For this review, take the finished solid that the model builds, in its own axes (mm). Face numbers are marked on the shaded views. A direction names the side the tool comes from. Coordinates: 2 decimals unless noted, no trailing zeros. Write each loop counter-clockwise with the first axis right and the second up, starting at its lowest first coordinate (ties: lowest second). Pieces come first, ordered by that corner, then holes. Notation, with made-up numbers: M 0.25,-15.75 L 19.25,-15.75 A31 cw 19.25,9.25 Z; hole C 51.5,-33 d4. An arc over 180 degrees is marked long. Return JSON: item names as keys, results as strings.
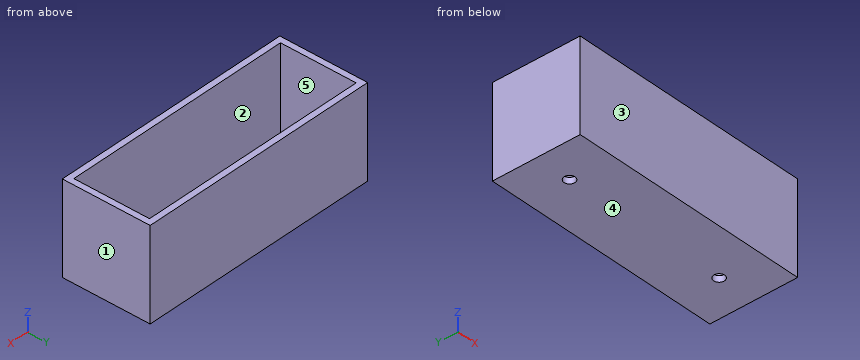
```python
from build123d import *

# Parameters (mm, degrees)
CYLINDER_R     = 1.8
CYLINDER_DEPTH = 50
ARRAY_X_COUNT  = 2
ARRAY_X_PITCH  = 55
BOX001_W       = 76
BOX001_H       = 25
BOX001_DEPTH   = 30
BOX_W          = 80
BOX_H          = 29
BOX_DEPTH      = 30


with BuildPart() as array:
    # Cylinder → Cylinder (new body)
    with BuildSketch(Plane(origin=(12.25, 14.5, -10), x_dir=(1, 0, 0), z_dir=(0, 0, 1))):
        Circle(CYLINDER_R)
    extrude(amount=CYLINDER_DEPTH)

    # Array X: Array ×2


with BuildPart() as array_1:
    add(array.part)
    with Locations(*[(i * ARRAY_X_PITCH, 0, 0) for i in range(1, ARRAY_X_COUNT)]):
        add(array.part)


with BuildPart() as fusion:
    # Box001 → Box001 (new body)
    with BuildSketch(Plane(origin=(2, 2, 2), x_dir=(1, 0, 0), z_dir=(0, 0, 1))):
        with Locations((38, 12.5)):
            Rectangle(BOX001_W, BOX001_H)
    extrude(amount=BOX001_DEPTH)

    # Fusion: union Array
    add(array_1.part)


with BuildPart() as cut:
    # Box → Box (new body)
    with BuildSketch(Plane.XY):
        with Locations((40, 14.5)):
            Rectangle(BOX_W, BOX_H)
    extrude(amount=BOX_DEPTH)

    # Cut: cut Fusion
    add(fusion.part, mode=Mode.SUBTRACT)


solid = cut.part
```
1. We need section D-D (x = 43). State the section outline as (y, z) points, plus the area to 3 significant figures.
Checks:
{"outline": "M 0,0 L 29,0 L 29,30 L 27,30 L 27,2 L 2,2 L 2,30 L 0,30 Z", "area": "170 mm2"}
2. Wall thickness on L1, parallel to X at y = 14.5, z = 1.15; L2, parallel to X at y = 6.5, z = 6.75; L3, parallel to Y at x = 53.5, z = 3: over which ranges is each line inside the solid? List them lowest first. Write a range as from..to.
Checks:
{"L1": "0..10.45, 14.05..65.45, 69.05..80", "L2": "0..2, 78..80", "L3": "0..2, 27..29"}
3. Clearance check with a flat-ended pin moving along its axis: pin 1 Ø1.5 at (x, y) = (56.5, 11) entering from +Z. State where the tip first meets the part, or that it passes through.
Checks:
{"pin 1": "z = 2"}
4. We need section A-A (z = 17). State the section outline as (x, y) points.
Checks:
{"outline": "M 0,0 L 80,0 L 80,29 L 0,29 Z; hole M 2,2 L 78,2 L 78,27 L 2,27 Z"}
5. We need section C-C (y = 19.5). State the section outline as (x, z) points.
Checks:
{"outline": "M 0,0 L 80,0 L 80,30 L 78,30 L 78,2 L 2,2 L 2,30 L 0,30 Z"}
6. We need section B-B (x = 12.25). State the section outline as (y, z) points.
Checks:
{"outline": "M 0,0 L 12.7,0 L 12.7,2 L 2,2 L 2,30 L 0,30 Z; M 16.3,0 L 29,0 L 29,30 L 27,30 L 27,2 L 16.3,2 Z"}
7. Draft analysis for pull direction Y (two halves, no side actions). For the marked faces 1, 2 and 3, state which applies: +Y half, -Y half, draft (parallel to the pull), parting line (faces both ways), or undercut.
Checks:
{"face 1": "draft", "face 2": "undercut", "face 3": "-Y half"}
8. For the marked faces 4 and 5, list the 3-axis set-ups (+Z, -Z, +X, -X, +Y, -Y) from which the entire face can be reached by the end or side of a thin tool; tool diameter is ignored.
Checks:
{"face 4": "-Z, +X, -X, +Y, -Y", "face 5": "+Z"}
